Here's the drawing with two shaded views (mm, measured from the low corner). I have some questions. A direction names the side the tool comes from. Coordinates: 2 decimals unless noted, no trailing zeros. Loops run counter-clockwise (first coordinate to the right, second up) from the corner with the lowest first, then second, coordinate; pieces in that order, holes last.
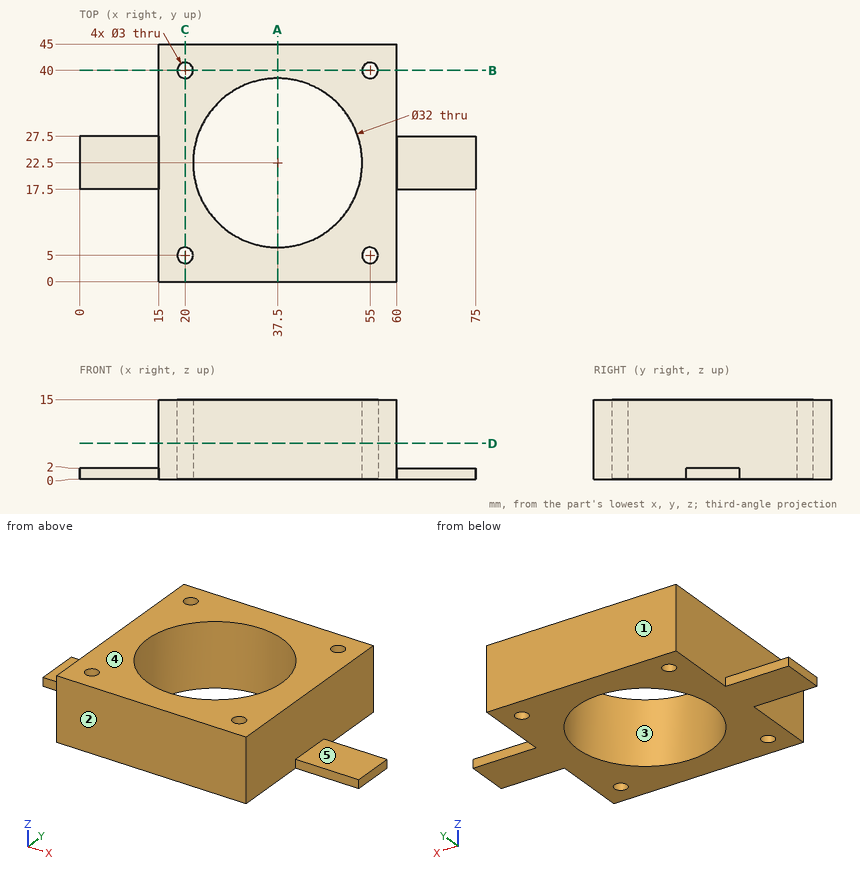
(1) I want a section at C-C on x = 20. Write out the boundary of the cut face in (y, z), then the cut area to 3 significant figures.
Check values:
outline: (0, 0) - (3.5, 0) - (3.5, 15) - (0, 15) - close; (6.5, 0) - (38.5, 0) - (38.5, 15) - (6.5, 15) - close; (41.5, 0) - (45, 0) - (45, 15) - (41.5, 15) - close
area: 585 mm2
(2) I'm going to push flat-ended pins straight in: pin 1 (4.5 mm diameter, centred on y = 30.5, z = 4, fed in from -X); pin 2 (3 mm diameter, centred on x = 66.5, y = 25, fed in from +Z); pin 3 (2 mm diameter, centred on x = 7.5, z = 0.5, fed in from +Y). Where does each tip first touch, or does it pass through?
Check values:
pin 1: stops at x = 15
pin 2: stops at z = 2
pin 3: stops at y = 27.5
(3) Which directions (+Z, -Z, +X, -X, +Y, -Y) give clear straight access to the entire face, cutting with the end or side of a thin tool? Please do the marked faces 4 and 5.
Check values:
face 4: +Z, +X, -X, +Y, -Y
face 5: +Z, +X, +Y, -Y
(4) I want a section at D-D on z = 6.75. Write out the boundary of the cut face in (x, y).
Check values:
outline: (15, 0) - (60, 0) - (60, 45) - (15, 45) - close; hole circle Ø3 at (20, 5); hole circle Ø3 at (20, 40); hole circle Ø32 at (37.5, 22.5); hole circle Ø3 at (55, 5); hole circle Ø3 at (55, 40)
(5) If we mould it in two halves opening along Y, with no side actions, what happens to the marked faces 1, 2 and 3? For each: released by +Y, released by -Y, zero draft, split by the parting line, or undercut.
Check values:
face 1: released by +Y
face 2: released by -Y
face 3: undercut
(6) I want a section at B-B on y = 40. Write out the boundary of the cut face in (x, z), then the cut area to 3 significant figures.
Check values:
outline: (15, 0) - (18.5, 0) - (18.5, 15) - (15, 15) - close; (21.5, 0) - (53.5, 0) - (53.5, 15) - (21.5, 15) - close; (56.5, 0) - (60, 0) - (60, 15) - (56.5, 15) - close
area: 585 mm2
(7) I want a section at A-A on x = 37.5. Write out the boundary of the cut face in (y, z).
Check values:
outline: (0, 0) - (6.5, 0) - (6.5, 15) - (0, 15) - close; (38.5, 0) - (45, 0) - (45, 15) - (38.5, 15) - close
(8) If I drill on probe 1 along Y at (x, z) = (55, 6.25); probe 2 along Y at (x, z) = (19, 7.25); probe 3 along X at (y, z) = (22, 12.25), over which ranges is the centre line in solid material (lowest first)?
Check values:
probe 1: y = 0 to 3.5, 6.5 to 38.5, 41.5 to 45
probe 2: y = 0 to 3.88, 6.12 to 38.88, 41.12 to 45
probe 3: x = 15 to 21.51, 53.49 to 60
